Geometry: final body of the model. Coordinates: model frame, mm. Face numbers are marked on the shaded views. A direction names the side the tool comes from. Round coordinates to 2 decimals unless told otherwise and drop trailing zeros. Loops run counter-clockwise (first coordinate to the right, second up) from the corner with the lowest first, then second, coordinate; pieces in that order, holes last. Notation, with made-up numbers: (15.5, 45) -> (62.5, 45) arc R20 cw to (62.5, 72) -> close; hole circle Ø2 at (86, -31). An arc over 180 degrees is marked (long way). Answer in a Markdown table with one row per item.
```python
from build123d import *

# Parameters (mm, degrees)
F1_DEPTH  = 40
F2_W      = 84
F2_H      = 36
F3_DEPTH  = 3
F4_T      = -2.5
F5_DEPTH  = 3
F7_DEPTH  = 3
F6_W      = 40
F6_H      = 40
F8_DEPTH  = 3
F9_DEPTH  = 0.2
F10_DEPTH = 0.5


with BuildPart() as f1:
    # F0 (on Front) → F1 (new body)
    with BuildSketch(Plane.XZ):
        Polygon((45, -3), (45, 3), (-45, 3), (-45, -3), (-20.5147061497, -3), (-20.5147061497, 0), (19.4852938503, 0), (19.4852938503, -3), align=None)
    extrude(amount=F1_DEPTH)

    # F2 (on face) → F3 (join)
    with BuildSketch(Plane.XY.offset(3)):
        with Locations((0.0693308115, -20.004203001)):
            Rectangle(F2_W, F2_H)
    extrude(amount=-F3_DEPTH)

    # F4
    f4_openings = [f1.faces().sort_by_distance(p)[0] for p in [
        (0, -20, 3),
    ]]
    offset(amount=F4_T, openings=f4_openings, kind=Kind.INTERSECTION)

    # F5 (cut): a face of the model
    f5_faces = [f1.faces().sort_by_distance(p)[0] for p in [
        (-0.5147061497, -20, 2.5),
    ]]
    extrude(f5_faces, amount=-F5_DEPTH, mode=Mode.SUBTRACT)

    # F7 (add): faces of the model
    f7_faces = [f1.faces().sort_by_distance(p)[0] for p in [
        (-32.7573530748, -20, -3),
        (32.2426469252, -20, -3),
    ]]
    extrude(f7_faces, amount=F7_DEPTH)

    # F6 (on Top) → F8 (join)
    with BuildSketch(Plane.XY):
        with Locations((-0.3256309032, -20)):
            Rectangle(F6_W, F6_H)
    extrude(amount=-F8_DEPTH)

    # F9 (add): a face of the model
    f9_faces = [f1.faces().sort_by_distance(p)[0] for p in [
        (-20.3256309032, -20, -1.5),
    ]]
    extrude(f9_faces, amount=F9_DEPTH)

    # F10 (add): faces of the model
    f10_faces = [f1.faces().sort_by_distance(p)[0] for p in [
        (-31.5128154516, -20, -0.5),
        (31.0871845484, -20, -0.5),
    ]]
    extrude(f10_faces, amount=F10_DEPTH)


solid = f1.part
```
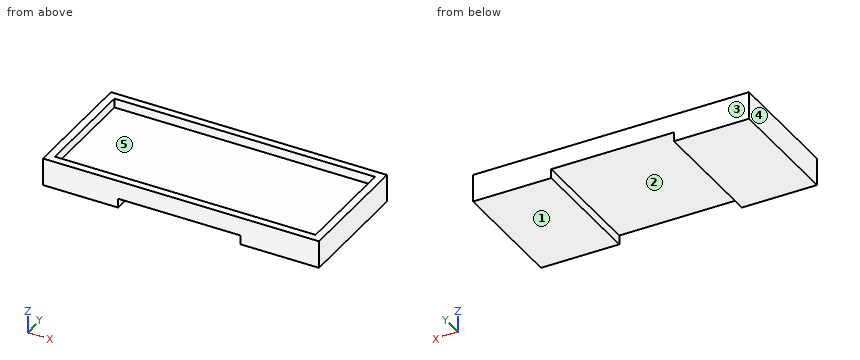
Item 1: Section query B-B, the plane x = -29. Output: boundary loops of the cut face in (y, z), and give its area (3 significant figures).
Ans:
| item | result |
|---|---|
| outline | (-40, -6) -> (0, -6) -> (0, 3) -> (-2.5, 3) -> (-2.5, 0) -> (-37.5, 0) -> (-37.5, 3) -> (-40, 3) -> close |
| area | 255 mm2 |
Item 2: Section query D-D, the plane y = -20.5. Output: boundary loops of the cut face in (x, z), and give its area (3 significant figures).
Ans:
| item | result |
|---|---|
| outline | (-45, -6) -> (-20.51, -6) -> (-20.51, -3) -> (19.49, -3) -> (19.49, -6) -> (45, -6) -> (45, 3) -> (42.5, 3) -> (42.5, 0) -> (-42.5, 0) -> (-42.5, 3) -> (-45, 3) -> close |
| area | 435 mm2 |
Item 3: First-contact query: P1, Ø10, axis at x = 35, y = -7, coming from the +Z side; P2, Ø5, axis at x = 1, y = -33, coming from the +Z side; P3, Ø20, axis at x = 7, y = -20.5, coming from the -Z side. Flat tips, straight axial feed; report the tip coordinate or a pass-through.
Ans:
| item | result |
|---|---|
| P1 | z = 3 |
| P2 | z = 0 |
| P3 | z = -3 |
Item 4: Set-up query: the marked faces 1 and 2. Return all of +Z, -Z, +X, -X, +Y, -Y with unobstructed straight access to the full face (end or side cutting, diameter ignored); none if empty.
Ans:
| item | result |
|---|---|
| face 1 | -Z, +X, -X, +Y, -Y |
| face 2 | -Z, +Y, -Y |
Item 5: Section query A-A, the plane z = -5. Output: boundary loops of the cut face in (x, y), and give its area (3 significant figures).
Ans:
| item | result |
|---|---|
| outline | (-45, -40) -> (-20.51, -40) -> (-20.51, 0) -> (-45, 0) -> close; (19.49, -40) -> (45, -40) -> (45, 0) -> (19.49, 0) -> close |
| area | 2,000 mm2 |
Item 6: Ray query, L1, parallel to Y at x = -0.5, z = 1; L2, parallel to X at y = -8, z = 0.25; L3, parallel to X at y = -22, z = -4.25. Return the intervals inside material, ascending.
Ans:
| item | result |
|---|---|
| L1 | -40 to -37.5, -2.5 to 0 |
| L2 | -45 to -42.5, 42.5 to 45 |
| L3 | -45 to -20.51, 19.49 to 45 |
Item 7: Mould query, pull axis Y, two halves, no side actions, for the marked faces 3, 4 and 5. Classes: released by +Y, released by -Y, zero draft, split by the parting line, or undercut.
Ans:
| item | result |
|---|---|
| face 3 | released by +Y |
| face 4 | zero draft |
| face 5 | undercut |
Item 8: Section query C-C, the plane z = 2. Output: boundary loops of the cut face in (x, y).
Ans:
| item | result |
|---|---|
| outline | (-45, -40) -> (45, -40) -> (45, 0) -> (-45, 0) -> close; hole (-42.5, -37.5) -> (42.5, -37.5) -> (42.5, -2.5) -> (-42.5, -2.5) -> close |
